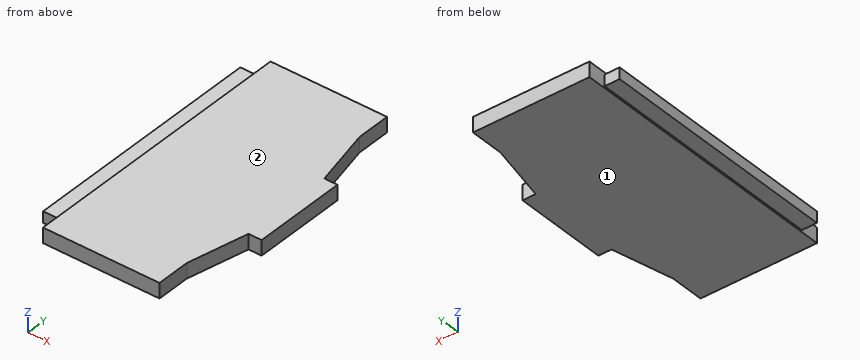
from build123d import *

# Parameters (mm, degrees)
BOSS_EXTRUDE1_DEPTH = 4
SKETCH3_W           = 3
SKETCH3_H           = 65
BOSS_EXTRUDE2_DEPTH = 4


with BuildPart() as part:
    # Sketch1 → Boss-Extrude1 (new body)
    with BuildSketch(Plane.XY):
        Polygon((0, 0), (31, 0), (31, 9), (34.5, 25), (38, 25), (38, 50), (34.5, 50), (31, 66), (31, 75), (0, 75), align=None)
    extrude(amount=BOSS_EXTRUDE1_DEPTH)

    # Sketch3 → Boss-Extrude2 (add)
    with BuildSketch(Plane.ZY):
        with Locations((2, 37.5)):
            Rectangle(SKETCH3_W, SKETCH3_H)
    extrude(amount=BOSS_EXTRUDE2_DEPTH)


solid = part.part
Read the model definition and answer for the solid it produces. Units are mm, in the model's axes. Face numbers are marked on the shaded views. Round coordinates to 2 decimals unless told otherwise and drop trailing zeros. Order: outer loops, then holes, each group sorted by start corner. A loop starts at its lowest first (then second) coordinate and runs counter-clockwise, first axis right, second up.
1) The mould has two halves that part along Z. Classify the marked faces 1 and 2: released by +Z, released by -Z, zero draft, split by the parting line, or undercut.
2) The part is cut by section D-D on y = 43.5. Write down the section's boundary in (x, z), plus the area to 3 significant figures.
3) Flat-ended cylindrical pins translate along their axes: pin 1 (3 mm diameter, centred on x = -2, y = 28.5, fed in from -Z); pin 2 (0.9 mm diameter, centred on x = -1.5, z = 2.5, fed in from +Y); pin 3 (1 mm diameter, centred on x = 35.5, z = 3, fed in from -Y). Find the tip coordinate at first contact, or state that the pin passes through.
4) The part is cut by section C-C on x = -1. Write down the section's boundary in (y, z).
5) Straight lines are drawn through the part: L1, parallel to Y at x = 36.5, z = 3.3; L2, parallel to X at y = 66, z = 2.95; L3, parallel to X at y = 16, z = 0.6. For each, find the intervals that lie inside material, in ascending order.
6) The part is cut by section B-B on z = 2.6. Write down the section's boundary in (x, y), plus the area to 3 significant figures.
7) The part is cut by section A-A on y = 6. Write down the section's boundary in (x, z).
Resolved:
1. face 1: released by -Z
1. face 2: released by +Z
2. outline: (-4, 0.5) - (0, 0.5) - (0, 0) - (38, 0) - (38, 4) - (0, 4) - (0, 3.5) - (-4, 3.5) - close
2. area: 164 mm2
3. pin 1: stops at z = 0.5
3. pin 2: stops at y = 70
3. pin 3: stops at y = 25
4. outline: (5, 0.5) - (70, 0.5) - (70, 3.5) - (5, 3.5) - close
5. L1: y = 25 to 50
5. L2: x = -4 to 31
5. L3: x = -4 to 32.53
6. outline: (-4, 5) - (0, 5) - (0, 0) - (31, 0) - (31, 9) - (34.5, 25) - (38, 25) - (38, 50) - (34.5, 50) - (31, 66) - (31, 75) - (0, 75) - (0, 70) - (-4, 70) - close
6. area: 2,820 mm2
7. outline: (-4, 0.5) - (0, 0.5) - (0, 0) - (31, 0) - (31, 4) - (0, 4) - (0, 3.5) - (-4, 3.5) - close
